Verification items for the finished model (mm, model axes). A direction names the side the tool comes from. Give positions to 0.01 mm unless a question says otherwise; leave off trailing zeros. Loops run counter-clockwise (first coordinate to the right, second up) from the corner with the lowest first, then second, coordinate; pieces in that order, holes last. Notation, with made-up numbers: (72.5, -16) - (104.5, -16) arc R29 cw to (104.5, 22) - close; hole circle Ø9 at (-17, -23.75). An arc over 180 degrees is marked (long way). Use one line per item in the form item = value.
```python
from build123d import *

# Parameters (mm, degrees)
SKETCH2_W                       = 90
SKETCH2_H                       = 90
BOSS_EXTRUDE1_DEPTH             = 6
SKETCH3_W                       = 6
SKETCH3_H                       = 90
BOSS_EXTRUDE2_DEPTH             = 75
SKETCH5_W                       = 90
SKETCH5_H                       = 6
BOSS_EXTRUDE3_DEPTH             = 16
SKETCH6_W                       = 90
SKETCH6_H                       = 6
BOSS_EXTRUDE4_DEPTH             = 16
CUT_EXTRUDE1_REACH              = 105.01
SKETCH7_R                       = 3
M5X0_8_TAPPED_HOLE2_D           = 4.2
M5X0_8_TAPPED_HOLE2_DEPTH       = 6
M5X0_8_TAPPED_HOLE2_CSINK_D     = 5.05
M5X0_8_TAPPED_HOLE2_CSINK_ANGLE = 100
FILLET2_R                       = 2


with BuildPart() as part:
    # Sketch2 → Boss-Extrude1 (new body)
    with BuildSketch(Plane(origin=(0, 0, 0), x_dir=(1, 0, 0), z_dir=(0, 1, 0))):
        Rectangle(SKETCH2_W, SKETCH2_H)
    extrude(amount=BOSS_EXTRUDE1_DEPTH)

    # Sketch3 → Boss-Extrude2 (add)
    with BuildSketch(Plane(origin=(0, 6, 0), x_dir=(1, 0, 0), z_dir=(0, 1, 0))):
        with Locations((-42, 0)):
            Rectangle(SKETCH3_W, SKETCH3_H)
        with Locations((42, 0)):
            Rectangle(SKETCH3_W, SKETCH3_H)
    extrude(amount=BOSS_EXTRUDE2_DEPTH)

    # Sketch5 → Boss-Extrude3 (add)
    with BuildSketch(Plane(origin=(-39, 0, 0), x_dir=(0, 0, -1), z_dir=(1, 0, 0))):
        with Locations((0, 72)):
            Rectangle(SKETCH5_W, SKETCH5_H)
    extrude(amount=BOSS_EXTRUDE3_DEPTH)

    # Sketch6 → Boss-Extrude4 (add)
    with BuildSketch(Plane.ZY.offset(-39)):
        with Locations((0, 72)):
            Rectangle(SKETCH6_W, SKETCH6_H)
    extrude(amount=BOSS_EXTRUDE4_DEPTH)

    # Sketch7 → Cut-Extrude1 (cut, up to next)
    with BuildSketch(Plane.XZ, mode=Mode.PRIVATE) as cut_extrude1_sk1:
        with Locations(Location((-25, 25, 0), (0, 0, 270))):
            Circle(SKETCH7_R)
    cut_extrude1_tool1 = extrude(cut_extrude1_sk1.sketch, amount=-CUT_EXTRUDE1_REACH, mode=Mode.PRIVATE) & part.part
    # Sketch7 → Cut-Extrude1 (cut, up to next)
    with BuildSketch(Plane.XZ, mode=Mode.PRIVATE) as cut_extrude1_sk2:
        with Locations(Location((25, 25, 0), (0, 0, 270))):
            Circle(SKETCH7_R)
    cut_extrude1_tool2 = extrude(cut_extrude1_sk2.sketch, amount=-CUT_EXTRUDE1_REACH, mode=Mode.PRIVATE) & part.part
    # Sketch7 → Cut-Extrude1 (cut, up to next)
    with BuildSketch(Plane.XZ, mode=Mode.PRIVATE) as cut_extrude1_sk3:
        with Locations(Location((25, -25, 0), (0, 0, 270))):
            Circle(SKETCH7_R)
    cut_extrude1_tool3 = extrude(cut_extrude1_sk3.sketch, amount=-CUT_EXTRUDE1_REACH, mode=Mode.PRIVATE) & part.part
    # Sketch7 → Cut-Extrude1 (cut, up to next)
    with BuildSketch(Plane.XZ, mode=Mode.PRIVATE) as cut_extrude1_sk4:
        with Locations(Location((-25, -25, 0), (0, 0, 270))):
            Circle(SKETCH7_R)
    cut_extrude1_tool4 = extrude(cut_extrude1_sk4.sketch, amount=-CUT_EXTRUDE1_REACH, mode=Mode.PRIVATE) & part.part
    add(cut_extrude1_tool1.solids().sort_by_distance((-25, 0, 25))[0], mode=Mode.SUBTRACT)
    add(cut_extrude1_tool2.solids().sort_by_distance((25, 0, 25))[0], mode=Mode.SUBTRACT)
    add(cut_extrude1_tool3.solids().sort_by_distance((25, 0, -25))[0], mode=Mode.SUBTRACT)
    add(cut_extrude1_tool4.solids().sort_by_distance((-25, 0, -25))[0], mode=Mode.SUBTRACT)

    # M5x0.8 Tapped Hole2
    with Locations(Plane(origin=(0, 75, 0), x_dir=(1, 0, 0), z_dir=(0, 1, 0))):
        with Locations((-28, 28), (-28, -28), (28, -28), (28, 28)):
            CounterSinkHole(M5X0_8_TAPPED_HOLE2_D / 2, M5X0_8_TAPPED_HOLE2_CSINK_D / 2, depth=M5X0_8_TAPPED_HOLE2_DEPTH, counter_sink_angle=M5X0_8_TAPPED_HOLE2_CSINK_ANGLE)

    # Fillet2
    fillet2_edges = [part.edges().sort_by_distance(p)[0] for p in [
        (-45, 40.5, 45),
        (-39, 37.5, 45),
        (0, 6, 45),
        (39, 37.5, 45),
        (45, 40.5, 45),
        (45, 40.5, -45),
        (39, 37.5, -45),
        (0, 6, -45),
        (-39, 37.5, -45),
        (-45, 40.5, -45),
        (39, 81, 0),
        (39, 6, 0),
        (-39, 6, 0),
        (-39, 81, 0),
    ]]
    fillet(fillet2_edges, radius=FILLET2_R)


solid = part.part
```
1. Section check A-A, the plane y = 25. Record the cut outline in (x, z), then the cut area to 3 significant figures.
Result set:
outline = (-45, -43) arc R2 ccw to (-43, -45) - (-41, -45) arc R2 ccw to (-39, -43) - (-39, 43) arc R2 ccw to (-41, 45) - (-43, 45) arc R2 ccw to (-45, 43) - close; (39, -43) arc R2 ccw to (41, -45) - (43, -45) arc R2 ccw to (45, -43) - (45, 43) arc R2 ccw to (43, 45) - (41, 45) arc R2 ccw to (39, 43) - close
area = 1,070 mm²
2. Depth check by flat-ended pin: pin 1 Ø5 at (x, z) = (-22, 8) entering from +Y; pin 2 Ø5.5 at (x, z) = (-30, -4) entering from -Y; pin 3 Ø2.5 at (x, z) = (28, -28) entering from +Y. Enter the tip coordinate at first touch or a pass-through.
Result set:
pin_1 = 75
pin_2 = 0
pin_3 = 6
3. Tool access check on faces 1 (the cylindrical face through (25, 3, -22)), 2 (the flat face through (-39, 77, 1)), 3 (the flat face through (-39, 38, 1)), 4 (the cylindrical face through (-25.9, 71.78, 27.91)), 5 (the flat face through (43, 81, -1)). Record the directions out of +Z, -Z, +X, -X, +Y, -Y that give a thin tool (end or side, any length) a straight path to the whole face; none if there is none.
Result set:
face_1 = -Y
face_2 = +Z, -Z, +Y
face_3 = +Z, -Z
face_4 = +Y
face_5 = +Z, -Z, +X, -X, +Y
4. Section check C-C, the plane z = -3. Record the cut outline in (x, y).
Result set:
outline = (-45, 0) - (45, 0) - (45, 81) - (41, 81) arc R2 ccw to (39, 79) - (39, 75) - (23, 75) - (23, 69) - (39, 69) - (39, 8) arc R2 cw to (37, 6) - (-37, 6) arc R2 cw to (-39, 8) - (-39, 69) - (-23, 69) - (-23, 75) - (-39, 75) - (-39, 79) arc R2 ccw to (-41, 81) - (-45, 81) - close
5. Section check B-B, the plane x = 35.5. Record the cut outline in (y, z), then the cut area to 3 significant figures.
Result set:
outline = (0, -45) - (4, -45) arc R2 ccw to (6, -43) - (6, 43) arc R2 ccw to (4, 45) - (0, 45) - close; (69, -45) - (75, -45) - (75, 45) - (69, 45) - close
area = 1,080 mm²
6. Scan lines: probe 1 along Z at (x, y) = (-28, 72); probe 2 along X at (y, z) = (2.95, -25); probe 3 along X at (y, z) = (70.2, -28). Record each from-to range of solid material in increasing order.
Result set:
probe_1 = -45 to -30.1, -25.9 to 25.9, 30.1 to 45
probe_2 = -45 to -28, -22 to 22, 28 to 45
probe_3 = -45 to -30.1, -25.9 to -23, 23 to 25.9, 30.1 to 45
7. Draft check along Z on faces 6 (the flat face through (45, 40, 1)), 7 (the cylindrical face through (30.1, 71.78, -28.09)), 8 (the cylindrical face through (30.1, 71.78, 27.91)), 9 (the flat face through (0, 1, -45)). Enter one of: released by +Z, released by -Z, zero draft, split by the parting line, or undercut.
Result set:
face_6 = zero draft
face_7 = undercut
face_8 = undercut
face_9 = released by -Z
8. Section check D-D, the plane x = 16. Record the cut outline in (y, z).
Result set:
outline = (0, -45) - (4, -45) arc R2 ccw to (6, -43) - (6, 43) arc R2 ccw to (4, 45) - (0, 45) - close
